```python
from build123d import *

# Parameters (mm, degrees)
SKETCH_W     = 100
SKETCH_H     = 50
PAD_DEPTH    = 2
SKETCH001_W  = 100
SKETCH001_H  = 25
PAD001_DEPTH = 31
SKETCH002_W  = 26
SKETCH002_H  = 28
POCKET_DEPTH = 100
CHAMFER_SIZE = 3
FILLET_R     = 3


with BuildPart() as part:
    # Sketch → Pad (new body)
    with BuildSketch(Plane.XY):
        Rectangle(SKETCH_W, SKETCH_H)
    extrude(amount=PAD_DEPTH)

    # Sketch001 (on Face6 of Pad) → Pad001 (join)
    with BuildSketch(Plane.XY.offset(2)):
        with Locations((0, -12.5)):
            Rectangle(SKETCH001_W, SKETCH001_H)
    extrude(amount=PAD001_DEPTH)

    # Sketch002 (on Face8 of Pad001) → Pocket (cut)
    with BuildSketch(Plane.YZ.offset(50)):
        with Locations((-9, 16)):
            Rectangle(SKETCH002_W, SKETCH002_H)
    extrude(amount=-POCKET_DEPTH, mode=Mode.SUBTRACT)

    # Chamfer
    chamfer_edges = [part.edges().sort_by_distance(p)[0] for p in [
        (0, -22, 2),
        (0, -22, 30),
    ]]
    chamfer(chamfer_edges, length=CHAMFER_SIZE)

    # Fillet
    fillet_edges = [part.edges().sort_by_distance(p)[0] for p in [
        (50, 25, 1),
        (-50, 25, 1),
        (-50, 0, 31.5),
        (50, 0, 31.5),
    ]]
    fillet(fillet_edges, radius=FILLET_R)


solid = part.part
```
The model under review builds one solid part; all positions refer to its coordinate system, in mm. A direction names the side the tool comes from. Round coordinates to 2 decimals unless told otherwise and drop trailing zeros. Loops run counter-clockwise (first coordinate to the right, second up) from the corner with the lowest first, then second, coordinate; pieces in that order, holes last. Notation, with made-up numbers: M 6,86.5 L 57,86.5 A9 ccw 57,92.5 Z; hole C 42.25,25 d2. An arc over 180 degrees is marked long. Answer as a JSON object with one key per item and string values.
(1) Take a section at A-A on y = -20.5. Give the boundary of the cut face in (x, z), and give its area (3 significant figures).
Resolved:
{"outline": "M -50,0 L 50,0 L 50,3.5 L -50,3.5 Z; M -50,28.5 L 50,28.5 L 50,33 L -50,33 Z", "area": "800 mm²"}
(2) Draft analysis for pull direction Z (two halves, no side actions). For faces 6 (the flat face through (-1, 0, 0)), 7 (the flat face through (1, -10, 30)), 8 (the cylindrical face through (49.1, 24.14, 1.01)), state which applies: released by +Z, released by -Z, zero draft, split by the parting line, or undercut.
Resolved:
{"face 6": "released by -Z", "face 7": "undercut", "face 8": "zero draft"}
(3) Take a section at B-B on x = 43. Give the boundary of the cut face in (y, z).
Resolved:
{"outline": "M -25,0 L 25,0 L 25,2 L -19,2 L -22,5 L -22,27 L -19,30 L 0,30 L 0,33 L -25,33 Z"}
(4) Take a section at D-D on z = 22.5. Give the boundary of the cut face in (x, y), and give its area (3 significant figures).
Resolved:
{"outline": "M -50,-25 L 50,-25 L 50,-22 L -50,-22 Z", "area": "300 mm²"}
(5) Tool access review of faces 1 (the cylindrical face through (-49.14, -0.9, 31.52)), 2 (the flat face through (-1, 3, 2)), 3 (the cylindrical face through (49.1, -0.86, 31.52)), 4 (the flat face through (-1, -12, 33)), 5 (the flat face through (-1, 0, 31)): name each direction out of +Z, -Z, +X, -X, +Y, -Y from which nothing blocks a thin tool from reaching the whole face with its end or side.
Resolved:
{"face 1": "+Z, -X, +Y", "face 2": "+X, -X, +Y", "face 3": "+Z, +X, +Y", "face 4": "+Z, +X, -X, +Y, -Y", "face 5": "+Z, +X, -X, +Y"}
(6) To check wall thickness, follow line 1 along Z through (x, y) = (-34, -2); line 2 along Z through (x, y) = (-44.5, 16); line 3 along Y through (x, z) = (9, 23). State the ranges of each line that lie inside material, in increasing order.
Resolved:
{"line 1": "0 to 2, 30 to 33", "line 2": "0 to 2", "line 3": "-25 to -22"}
(7) Take a section at C-C on y = -8.5. Give the boundary of the cut face in (x, z).
Resolved:
{"outline": "M -50,0 L 50,0 L 50,2 L -50,2 Z; M -50,30 L 50,30 L 50,33 L -50,33 Z"}
(8) Clearance check with flat-ended pins moving along their axes: P1, Ø1.5, axis at x = -5, z = 31, coming from the +Y side; P2, Ø13, axis at x = 12.5, y = 11, coming from the +Z side; P3, Ø4, axis at x = -4.5, y = 8, coming from the -Z side; P4, Ø8, axis at x = -38.5, z = 23.5, coming from the +Y side. State where each tip first meets the part, or that it passes through.
Resolved:
{"P1": "y = 0", "P2": "z = 2", "P3": "z = 0", "P4": "y = -21.5"}
